For this review, take the finished solid that the model builds, in its own axes (mm). Face numbers are marked on the shaded views. A direction names the side the tool comes from. Coordinates: 2 decimals unless noted, no trailing zeros. Order: outer loops, then holes, each group sorted by start corner. A loop starts at its lowest first (then second) coordinate and runs counter-clockwise, first axis right, second up. Notation, with made-up numbers: (-10.5, 9.25) -> (16.5, 9.25) arc R21 ccw to (16.5, 24.25) -> close; hole circle Ø2 at (-29.75, 12.5). An arc over 180 degrees is marked (long way). Write item = value, one per line. Start each with the question number.
1) Consider section A-A on y = 0. Give the boundary of the cut face in (x, z) (1 decimal).
2) Insertion check: pin 1 Ø12 at (x, z) = (11, -11) entering from -Y; pin 2 Ø3 at (y, z) = (-8.5, 5) entering from +X; pin 3 Ø12 at (y, z) = (6.5, -1) entering from -X; pin 4 Ø4 at (y, z) = (0, 0) entering from -X. Each pin has a flat end and moves straight along its axis. Give the tip position at first contact, or say it passes through.
3) Consider section D-D on z = -3.75. Give the boundary of the cut face in (x, y) (1 decimal).
4) Machinability: for the marked faces 1, 2 and 3, which of the approach directions +Z, -Z, +X, -X, +Y, -Y give a long, thin tool a straight path to every point of the face, cutting with its end or side? Answer none if there is none.
5) Wall thickness on probe 1 along Y at (x, z) = (20.25, 0); probe 2 along Z at (x, y) = (6, 7.5); probe 3 along X at (y, z) = (13, 3): over which ranges is each line inside the solid? List them lowest first. Write a range as [from, to].
6) Draft analysis for pull direction Z (two halves, no side actions). For the marked faces 4, 5 and 6, state which applies: +Z half, -Z half, draft (parallel to the pull), parting line (faces both ways), or undercut.
7) Consider section C-C on x = 8. Give the boundary of the cut face in (y, z) (3 decimals).
Autodesk Inventor part; units mm, degrees
ref_plane "YZ Plane" through (0, 0, 0) normal (1, 0, 0) x (0, 1, 0)
ref_plane "XZ Plane" through (0, 0, 0) normal (0, 1, 0) x (-1, 0, 0)
ref_plane "XY Plane" through (0, 0, 0) normal (0, 0, 1) x (1, 0, 0)
sketch "Sketch3" plane through (0, 0, 0) normal (1, 0, 0) x (0, 1, 0)
  circle A0 centre (0, 0) radius 15.875 construction
  circle A1 centre (0, 0) radius 14.6304
  dimension "d8" = 31.75
  dimension "d9" = 1.2446
extrude "Extrusion3" add sketch "Sketch3" along normal blind 12.7
sketch "Sketch4" plane through (12.7, 0, 0) normal (1, 0, 0) x (0, 0, -1)
  circle A0 centre (0, 0) radius 4.7625
  dimension "d12" = 9.525
extrude "Extrusion4" add sketch "Sketch4" along normal blind 17.4625
sketch "Sketch5" plane through (30.1625, 0, 0) normal (1, 0, 0) x (0, 0, -1)
  circle A0 centre (0, 0) radius 2.4892
  dimension "d15" = 4.9784
extrude "Extrusion5" cut sketch "Sketch5" against normal through all
sketch "Sketch6" plane through (0, 0, 0) normal (-1, 0, 0) x (0, 0, 1)
  circle A0 centre (0, 0) radius 9.525
  dimension "d18" = 19.05
extrude "Extrusion6" cut sketch "Sketch6" against normal blind 9.525
properties part number "Long roller plug 2"
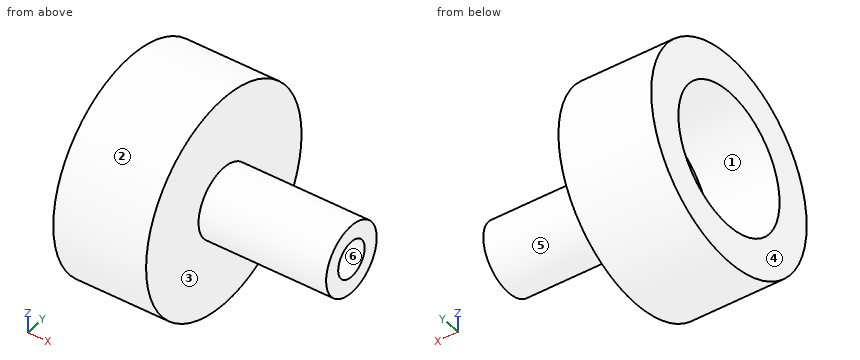
Answer sheet:
q1.outline = (0, -14.6) -> (12.7, -14.6) -> (12.7, -4.8) -> (30.2, -4.8) -> (30.2, -2.5) -> (9.5, -2.5) -> (9.5, -9.5) -> (0, -9.5) -> close; (0, 9.5) -> (9.5, 9.5) -> (9.5, 2.5) -> (30.2, 2.5) -> (30.2, 4.8) -> (12.7, 4.8) -> (12.7, 14.6) -> (0, 14.6) -> close
q2.pin_1 = -13.75
q2.pin_2 = 12.7
q2.pin_3 = 0
q2.pin_4 = through
q3.outline = (0, -14.1) -> (12.7, -14.1) -> (12.7, -2.9) -> (30.2, -2.9) -> (30.2, 2.9) -> (12.7, 2.9) -> (12.7, 14.1) -> (0, 14.1) -> (0, 8.8) -> (9.5, 8.8) -> (9.5, -8.8) -> (0, -8.8) -> close
q4.face_1 = -X
q4.face_2 = +X, -X
q4.face_3 = +X
q5.probe_1 = [-4.76, -2.49], [2.49, 4.76]
q5.probe_2 = [-12.56, -5.87], [5.87, 12.56]
q5.probe_3 = [0, 12.7]
q6.face_4 = draft
q6.face_5 = parting line
q6.face_6 = undercut
q7.outline = circle Ø29.261 at (0, 0); hole circle Ø19.05 at (0, 0)
